Read the model definition and answer for the solid it produces. Units are mm, in the model's axes. Face numbers are marked on the shaded views. A direction names the side the tool comes from. Give positions to 0.01 mm unless a question says otherwise; leave off trailing zeros. Write each question's results on one line, items separated by ' | '. Start each with the question number.
Item 1: This flat-tipped pin is pushed along its axis until it touches: P1, Ø2, axis at x = 4, y = 3.5, coming from the +Z side. Where does it stop, or does it pass through?
Item 2: Which of the six approach directions +Z, -Z, +X, -X, +Y, -Y give full straight-line access (tool end or side, diameter ignored) to the marked faces 1, 2 and 3?
Item 3: Find the intervals of material crossed by line 1 (X direction, y = -3.5, z = 14.5); line 2 (Y direction, x = 4.25, z = 5); line 3 (Z direction, x = 3.75, y = 7.25), in increasing order.
Item 4: Section A-A on z = 21 is taken. State how many separate pieces and enclosed holes the cut face has, and give its area (3 significant figures).
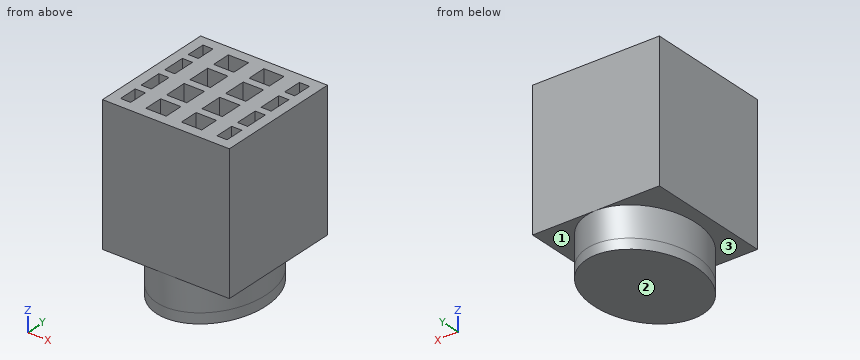
```python
from build123d import *

# Parameters (mm, degrees)
SKETCH_8_W       = 25
SKETCH_8_H       = 25
SKETCH_8_W_2     = 4
SKETCH_8_H_2     = 21
SKETCH_8_W_3     = 2
EXTRUDE_7_DEPTH  = 25
SKETCH_9_W       = 25
SKETCH_9_H       = 25
EXTRUDE_8_DEPTH  = 2
SKETCH_14_W      = 25
SKETCH_14_H      = 1.5
EXTRUDE_11_DEPTH = 25
SKETCH_16_RX     = 12.5
SKETCH_16_RY     = 10
SKETCH_16_RX_2   = 10.5
SKETCH_16_RY_2   = 8
EXTRUDE_14_DEPTH = 6
SKETCH_22_RX     = 12.5
SKETCH_22_RY     = 10
EXTRUDE_18_DEPTH = 2


with BuildPart() as part:
    # 草图8 → 凸台-拉伸7 (new body)
    with BuildSketch(Plane.XY):
        Rectangle(SKETCH_8_W, SKETCH_8_H)
        with Locations((3.5, 0)):
            Rectangle(SKETCH_8_W_2, SKETCH_8_H_2, mode=Mode.SUBTRACT)
        with Locations((-3.5, 0)):
            Rectangle(SKETCH_8_W_2, SKETCH_8_H_2, mode=Mode.SUBTRACT)
        with Locations((-9.5, 0)):
            Rectangle(SKETCH_8_W_3, SKETCH_8_H_2, mode=Mode.SUBTRACT)
        with Locations((9.5, 0)):
            Rectangle(SKETCH_8_W_3, SKETCH_8_H_2, mode=Mode.SUBTRACT)
    extrude(amount=EXTRUDE_7_DEPTH)

    # 草图9 → 凸台-拉伸8 (add)
    with BuildSketch(Plane(origin=(0, 0, 0), x_dir=(-1, 0, 0), z_dir=(0, 0, -1))):
        Rectangle(SKETCH_9_W, SKETCH_9_H)
    extrude(amount=EXTRUDE_8_DEPTH)

    # 草图14 → 凸台-拉伸11 (add)
    with BuildSketch(Plane.XY.offset(25)):
        Rectangle(SKETCH_14_W, SKETCH_14_H)
        with Locations((0, 6)):
            Rectangle(SKETCH_14_W, SKETCH_14_H)
        with Locations((0, -6)):
            Rectangle(SKETCH_14_W, SKETCH_14_H)
    extrude(amount=-EXTRUDE_11_DEPTH)

    # 草图16 → 凸台-拉伸14 (add)
    with BuildSketch(Plane(origin=(0, 0, -2), x_dir=(-1, 0, 0), z_dir=(0, 0, -1))):
        with Locations(Location((0, 0), (0, 0, -90))):
            Ellipse(SKETCH_16_RX, SKETCH_16_RY)
        with Locations(Location((0, 0), (0, 0, -90))):
            Ellipse(SKETCH_16_RX_2, SKETCH_16_RY_2, mode=Mode.SUBTRACT)
    extrude(amount=EXTRUDE_14_DEPTH)

    # 草图22 → 凸台-拉伸18 (add)
    with BuildSketch(Plane(origin=(0, 0, -8), x_dir=(-1, 0, 0), z_dir=(0, 0, -1))):
        with Locations(Location((0, 0), (0, 0, -90))):
            Ellipse(SKETCH_22_RX, SKETCH_22_RY)
    extrude(amount=EXTRUDE_18_DEPTH)


solid = part.part
```
Findings:
1) P1: z = 0
2) face 1: -Z, +X | face 2: -Z, +X, -X, +Y, -Y | face 3: -Z, -X
3) line 1: -12.5 to -10.5, -8.5 to -5.5, -1.5 to 1.5, 5.5 to 8.5, 10.5 to 12.5 | line 2: -12.5 to -10.5, -6.75 to -5.25, -0.75 to 0.75, 5.25 to 6.75, 10.5 to 12.5 | line 3: -10 to -8, -2 to 0
4) separate pieces: 1 | enclosed holes: 16 | area: 427 mm2
